Input: part model. Units: mm. Frame: model coordinates. Face numbers are marked on the shaded views. A direction names the side the tool comes from. Round coordinates to 2 decimals unless told otherwise and drop trailing zeros. Order: outer loops, then holes, each group sorted by start corner. A loop starts at its lowest first (then second) coordinate and runs counter-clockwise, first axis right, second up. Notation, with made-up numbers: (-38.75, -11.75) - (-1.75, -11.75) arc R22 cw to (-1.75, 3.25) - close; hole circle Ø3 at (32, 52). An arc over 180 degrees is marked (long way). One line per item, written item: value. Start each with the question number.
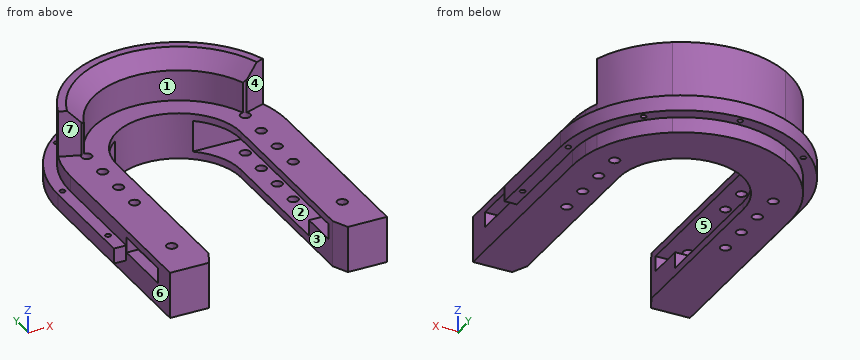
from build123d import *

# Parameters (mm, degrees)
BOSS_EXTRUDE1_DEPTH     = 30
CUT_EXTRUDE1_START      = 5
CUT_EXTRUDE1_DEPTH      = 20.4
SKETCH3_R               = 3.275
CUT_EXTRUDE2_DEPTH      = 139.032749737
LPATTERN1_COUNT         = 4
LPATTERN1_PITCH         = 20
CUT_EXTRUDE3_START      = -4.6
CUT_EXTRUDE3_DEPTH      = 10
SKETCH5_R               = 3.275
CUT_EXTRUDE4_DEPTH      = 17.6
BOSS_EXTRUDE2_DEPTH     = 30
MIRROR1_COPY_1_SKETCH_R = 3.275
MIRROR1_COPY_1_DEPTH    = 139.032749737
MIRROR1_COPY_2_SKETCH_R = 3.275
MIRROR1_COPY_2_DEPTH    = 139.032749737
MIRROR1_COPY_3_SKETCH_R = 3.275
MIRROR1_COPY_3_DEPTH    = 139.032749737
BOSS_EXTRUDE3_START     = 30
BOSS_EXTRUDE3_DEPTH     = 30
CUT_EXTRUDE5_REACH      = 148.469
BOSS_EXTRUDE4_DEPTH     = 30
BOSS_EXTRUDE5_DEPTH     = 5
CHAMFER1_SIZE           = 10
SKETCH11_R              = 1.7
CUT_EXTRUDE6_DEPTH      = 10


with BuildPart() as part:
    # Sketch1 → Boss-Extrude1 (new body)
    with BuildSketch(Plane.XY):
        with BuildLine():
            Line((70.2, 60), (-70.2, 60))
            Line((-70.2, 60), (-70.2, -115))
            Line((-70.2, -115), (-40.2, -115))
            Line((-40.2, -115), (-40.2, 0))
            ThreePointArc((-40.2, 0), (0, 40.2), (40.2, 0))
            Line((40.2, 0), (40.2, -115))
            Line((40.2, -115), (70.2, -115))
            Line((70.2, -115), (70.2, 60))
        make_face()
    extrude(amount=BOSS_EXTRUDE1_DEPTH)

    # Sketch2 → Cut-Extrude1 (cut)
    with BuildSketch(Plane.XY.offset(CUT_EXTRUDE1_START)):
        Polygon((25.2, 31.320919527), (25.2, -45), (40.2, -60), (40.2, -85.4), (62.5, -85.4), (62.5, 31.320919527), align=None)
    cut_extrude1 = extrude(amount=CUT_EXTRUDE1_DEPTH, mode=Mode.SUBTRACT)

    # Sketch3 → Cut-Extrude2 (cut, through all)
    with BuildSketch(Plane.XY.offset(30)):
        with Locations((51.35, 16.120919527)):
            Circle(SKETCH3_R)
    cut_extrude2 = extrude(amount=-CUT_EXTRUDE2_DEPTH, mode=Mode.SUBTRACT)

    # LPattern1: Cut-Extrude2 ×4
    with Locations(*[(0, -i * LPATTERN1_PITCH, 0) for i in range(1, LPATTERN1_COUNT)]):
        add(cut_extrude2, mode=Mode.SUBTRACT)

    # Sketch6 → Cut-Extrude3 (cut)
    with BuildSketch(Plane.XY.offset(30).offset(CUT_EXTRUDE3_START)):
        Polygon((40.2, -85.4), (55.2, -85.4), (55.2, -70.4), (70.2, -70.4), (70.2, -110), (40.2, -110), align=None)
    cut_extrude3 = extrude(amount=-CUT_EXTRUDE3_DEPTH, mode=Mode.SUBTRACT)

    # Sketch5 → Cut-Extrude4 (cut)
    with BuildSketch(Plane.XY.offset(30)):
        with Locations((55.2, -98)):
            Circle(SKETCH5_R)
    cut_extrude4 = extrude(amount=-CUT_EXTRUDE4_DEPTH, mode=Mode.SUBTRACT)

    # Sketch7 → Boss-Extrude2 (add)
    with BuildSketch(Plane.XY.offset(30)):
        Polygon((40.2, -115), (70.2, -115), (70.2, -125), (44.863076582, -125), align=None)
    boss_extrude2 = extrude(amount=-BOSS_EXTRUDE2_DEPTH)

    # Mirror1: Cut-Extrude1, Cut-Extrude2, Cut-Extrude3, Cut-Extrude4, Boss-Extrude2 across plane
    add(cut_extrude1.mirror(Plane(origin=(0, 0, 0), x_dir=(0, 0, 1), z_dir=(1, 0, 0))), mode=Mode.SUBTRACT)
    add(cut_extrude2.mirror(Plane(origin=(0, 0, 0), x_dir=(0, 0, 1), z_dir=(1, 0, 0))), mode=Mode.SUBTRACT)
    add(cut_extrude3.mirror(Plane(origin=(0, 0, 0), x_dir=(0, 0, 1), z_dir=(1, 0, 0))), mode=Mode.SUBTRACT)
    add(cut_extrude4.mirror(Plane(origin=(0, 0, 0), x_dir=(0, 0, 1), z_dir=(1, 0, 0))), mode=Mode.SUBTRACT)
    add(boss_extrude2.mirror(Plane(origin=(0, 0, 0), x_dir=(0, 0, 1), z_dir=(1, 0, 0))))

    # Mirror1 copy 1 sketch → Mirror1 copy 1 (cut, through all)
    with BuildSketch(Plane(origin=(0, -20, 30), x_dir=(-1, 0, 0), z_dir=(0, 0, 1))):
        with Locations((51.35, -16.120919527)):
            Circle(MIRROR1_COPY_1_SKETCH_R)
    extrude(amount=-MIRROR1_COPY_1_DEPTH, mode=Mode.SUBTRACT)

    # Mirror1 copy 2 sketch → Mirror1 copy 2 (cut, through all)
    with BuildSketch(Plane(origin=(0, -40, 30), x_dir=(-1, 0, 0), z_dir=(0, 0, 1))):
        with Locations((51.35, -16.120919527)):
            Circle(MIRROR1_COPY_2_SKETCH_R)
    extrude(amount=-MIRROR1_COPY_2_DEPTH, mode=Mode.SUBTRACT)

    # Mirror1 copy 3 sketch → Mirror1 copy 3 (cut, through all)
    with BuildSketch(Plane(origin=(0, -60, 30), x_dir=(-1, 0, 0), z_dir=(0, 0, 1))):
        with Locations((51.35, -16.120919527)):
            Circle(MIRROR1_COPY_3_SKETCH_R)
    extrude(amount=-MIRROR1_COPY_3_DEPTH, mode=Mode.SUBTRACT)

    # Sketch8 → Boss-Extrude3 (add)
    with BuildSketch(Plane.XY.offset(30).offset(BOSS_EXTRUDE3_START)):
        with BuildLine():
            ThreePointArc((51.467268944, 19.393819311), (52.549226062, 19.168456541), (53.494616948, 18.596044401))
            Line((53.494616948, 18.596044401), (66.307819698, 23.050228782))
            ThreePointArc((66.307819698, 23.050228782), (54.595945877, 44.128479395), (36.442283134, 60))
            Line((36.442283134, 60), (-36.442283134, 60))
            ThreePointArc((-36.442283134, 60), (-54.595945877, 44.128479395), (-66.307819698, 23.050228782))
            Line((-66.307819698, 23.050228782), (-53.494616948, 18.596044401))
            ThreePointArc((-53.494616948, 18.596044401), (-52.549226062, 19.168456541), (-51.467268944, 19.393819311))
            ThreePointArc((-51.467268944, 19.393819311), (0, 55), (51.467268944, 19.393819311))
        make_face()
        with BuildLine():
            Line((-36.442283134, 60), (36.442283134, 60))
            ThreePointArc((36.442283134, 60), (0, 70.2), (-36.442283134, 60))
        make_face()
    extrude(amount=-BOSS_EXTRUDE3_DEPTH)

    # Sketch8<3> → Cut-Extrude5 (cut, up to next)
    with BuildSketch(Plane.XY.offset(30), mode=Mode.PRIVATE) as cut_extrude5_sk1:
        with BuildLine():
            Line((-70.2, 24.403246372), (-66.307819698, 23.050228782))
            ThreePointArc((-66.307819698, 23.050228782), (-54.595945877, 44.128479395), (-36.442283134, 60))
            Line((-36.442283134, 60), (-70.2, 60))
            Line((-70.2, 60), (-70.2, 24.403246372))
        make_face()
    cut_extrude5_tool1 = extrude(cut_extrude5_sk1.sketch, amount=-CUT_EXTRUDE5_REACH, mode=Mode.PRIVATE) & part.part
    # Sketch8<3> → Cut-Extrude5 (cut, up to next)
    with BuildSketch(Plane.XY.offset(30), mode=Mode.PRIVATE) as cut_extrude5_sk2:
        with BuildLine():
            ThreePointArc((36.442283134, 60), (54.595945877, 44.128479395), (66.307819698, 23.050228782))
            Line((66.307819698, 23.050228782), (70.2, 24.403246372))
            Line((70.2, 24.403246372), (70.2, 60))
            Line((70.2, 60), (36.442283134, 60))
        make_face()
    cut_extrude5_tool2 = extrude(cut_extrude5_sk2.sketch, amount=-CUT_EXTRUDE5_REACH, mode=Mode.PRIVATE) & part.part
    # Sketch8<3> → Cut-Extrude5 (cut, up to next)
    with BuildSketch(Plane.XY.offset(30), mode=Mode.PRIVATE) as cut_extrude5_sk3:
        with BuildLine():
            ThreePointArc((-70.2, -2.11e-07), (-69.220116107, 11.688264463), (-66.307819698, 23.050228782))
            Line((-66.307819698, 23.050228782), (-70.2, 24.403246372))
            Line((-70.2, 24.403246372), (-70.2, -2.11e-07))
        make_face()
    cut_extrude5_tool3 = extrude(cut_extrude5_sk3.sketch, amount=-CUT_EXTRUDE5_REACH, mode=Mode.PRIVATE) & part.part
    # Sketch8<3> → Cut-Extrude5 (cut, up to next)
    with BuildSketch(Plane.XY.offset(30), mode=Mode.PRIVATE) as cut_extrude5_sk4:
        with BuildLine():
            Line((70.2, 24.403246372), (66.307819698, 23.050228782))
            ThreePointArc((66.307819698, 23.050228782), (67.781169893, 18.268908232), (68.910228278, 13.394791475))
            ThreePointArc((68.910228278, 13.394791475), (69.876813125, 6.728371827), (70.2, 0))
            Line((70.2, 0), (70.2, 24.403246372))
        make_face()
    cut_extrude5_tool4 = extrude(cut_extrude5_sk4.sketch, amount=-CUT_EXTRUDE5_REACH, mode=Mode.PRIVATE) & part.part
    add(cut_extrude5_tool1.solids().sort_by_distance((-60.211924, 47.421262, 30))[0], mode=Mode.SUBTRACT)
    add(cut_extrude5_tool2.solids().sort_by_distance((60.211924, 47.421262, 30))[0], mode=Mode.SUBTRACT)
    add(cut_extrude5_tool3.solids().sort_by_distance((-69.027031, 17.825577, 30))[0], mode=Mode.SUBTRACT)
    add(cut_extrude5_tool4.solids().sort_by_distance((69.027031, 17.825577, 30))[0], mode=Mode.SUBTRACT)

    # Sketch8<4> → Boss-Extrude4 (add)
    with BuildSketch(Plane.XY.offset(30)):
        with BuildLine():
            Line((-36.442283134, 60), (36.442283134, 60))
            ThreePointArc((36.442283134, 60), (0, 70.2), (-36.442283134, 60))
        make_face()
    extrude(amount=-BOSS_EXTRUDE4_DEPTH)

    # Sketch10 → Boss-Extrude5 (add, symmetric)
    with BuildSketch(Plane.XY.offset(15)):
        with BuildLine():
            Line((78.2, 0), (78.2, -70))
            Line((78.2, -70), (70.2, -70))
            Line((70.2, -70), (70.2, 0))
            ThreePointArc((70.2, 0), (69.220116089, 11.688264568), (66.307819698, 23.050228782))
            ThreePointArc((66.307819698, 23.050228782), (0, 70.2), (-66.307819698, 23.050228782))
            ThreePointArc((-66.307819698, 23.050228782), (-69.220116089, 11.688264568), (-70.2, 0))
            Line((-70.2, 0), (-70.2, -70))
            Line((-70.2, -70), (-78.2, -70))
            Line((-78.2, -70), (-78.2, 0))
            ThreePointArc((-78.2, 0), (-77.108448407, 13.02026053), (-73.864266387, 25.677035481))
            ThreePointArc((-73.864266387, 25.677035481), (0, 78.2), (73.864266387, 25.677035481))
            ThreePointArc((73.864266387, 25.677035481), (77.108448407, 13.02026053), (78.2, 0))
        make_face()
    extrude(amount=BOSS_EXTRUDE5_DEPTH, both=True)

    # Chamfer1
    chamfer1_edges = [part.edges().sort_by_distance(p)[0] for p in [
        (0, 55, 60),
    ]]
    chamfer(chamfer1_edges, length=CHAMFER1_SIZE)

    # Sketch11 → Cut-Extrude6 (cut)
    with BuildSketch(Plane.XY.offset(20)):
        with Locations((-74.2, -55)):
            Circle(SKETCH11_R)
        with Locations((-74.167849765, 2.184046985)):
            Circle(SKETCH11_R)
        with Locations((-51.689378569, 53.233900319)):
            Circle(SKETCH11_R)
        with Locations((0, 74.2)):
            Circle(SKETCH11_R)
        with Locations((51.689378569, 53.233900319)):
            Circle(SKETCH11_R)
        with Locations((74.167849765, 2.184046985)):
            Circle(SKETCH11_R)
        with Locations((74.2, -55)):
            Circle(SKETCH11_R)
    extrude(amount=-CUT_EXTRUDE6_DEPTH, mode=Mode.SUBTRACT)


solid = part.part
Item 1: Section query B-B on y = -12.5. Return loops of the section in (x, z), and give its area (3 significant figures).
Item 2: Pull-direction query (Y, two-part tool) for the marked faces 5, 6 and 7; classes: released by +Y, released by -Y, zero draft, split by the parting line, or undercut.
Item 3: First-contact query: pin 1 Ø5 at (x, z) = (57.5, 22) entering from +Y; pin 2 Ø5 at (x, y) = (-42.5, -7.5) entering from +Z; pin 3 Ø5.5 at (x, y) = (74.17, 2.18) entering from +Z. Flat tips, straight axial feed; report the tip coordinate or a pass-through.
Item 4: Reachability of the marked faces 1, 2, 3 and 4 from +Z, -Z, +X, -X, +Y, -Y: full face, straight path, thin tool, end or side. Return the list, or none.
Item 5: Section query A-A on y = -98. Give the number of separate pieces and of enclosed holes in the cut face, and give its area (3 significant figures).
Item 6: Line query: L1, parallel to X at y = -62.5, z = 8; L2, parallel to Z at x = 65.5, y = -84; L3, parallel to X at y = -73.5, z = 27. Output: solid intervals per line, ascending.
Geometry results:
1. outline: (-78.2, 10) - (-70.2, 10) - (-70.2, 0) - (-40.2, 0) - (-40.2, 5) - (-62.5, 5) - (-62.5, 25.4) - (-40.2, 25.4) - (-40.2, 30) - (-70.2, 30) - (-70.2, 20) - (-78.2, 20) - close; (40.2, 0) - (70.2, 0) - (70.2, 10) - (78.2, 10) - (78.2, 20) - (70.2, 20) - (70.2, 30) - (40.2, 30) - (40.2, 25.4) - (62.5, 25.4) - (62.5, 5) - (40.2, 5) - close
1. area: 1,050 mm^2
2. face 5: undercut
2. face 6: zero draft
2. face 7: released by -Y
3. pin 1: stops at y = 54.58
3. pin 2: stops at z = 30
3. pin 3: stops at z = 20
4. face 1: +Z, -Y
4. face 2: none
4. face 3: +Z, -Z, -Y
4. face 4: +Z, +X, -Y
5. separate pieces: 6
5. enclosed holes: 0
5. area: 1,100 mm^2
6. L1: x = -70.2 to -62.5, 62.5 to 70.2
6. L2: z = 0 to 15.4, 25.4 to 30
6. L3: x = -70.2 to -40.2, 40.2 to 70.2
